```python
from build123d import *

# Parameters (mm, degrees)
F1_DEPTH = 39.6875
F2_W     = 152.4
F2_H     = 25.4
F3_DEPTH = 42.8625
F4_W     = 152.4
F4_H     = 13.716
F5_DEPTH = 42.8498


with BuildPart() as f1:
    # F0 (on Front) → F1 (new body)
    with BuildSketch(Plane.XZ):
        with BuildLine():
            Line((0, 25.4), (0, 0))
            Line((0, 0), (34.078865, 0))
            ThreePointArc((34.078865, 0), (76.2, 12.7), (118.321135, 0))
            Line((118.321135, 0), (152.4, 0))
            Line((152.4, 0), (152.4, 25.4))
            Line((152.4, 25.4), (0, 25.4))
        make_face()
    extrude(amount=F1_DEPTH)

    # F2 (on face) → F3 (join)
    with BuildSketch(Plane(origin=(0, 0, 0), x_dir=(-1, 0, 0), z_dir=(0, 1, 0))):
        with Locations((-76.2, 12.7)):
            Rectangle(F2_W, F2_H)
    extrude(amount=F3_DEPTH)

    # F4 (on face) → F5 (cut)
    with BuildSketch(Plane(origin=(0, 42.8625, 0), x_dir=(-1, 0, 0), z_dir=(0, 1, 0))):
        with Locations((-76.2, 18.542)):
            Rectangle(F4_W, F4_H)
    extrude(amount=-F5_DEPTH, mode=Mode.SUBTRACT)


solid = f1.part
```
The listing builds one solid part. Answer for the finished solid, in the listing's coordinates (mm). A direction names the side the tool comes from. Give positions to 0.01 mm unless a question says otherwise; leave off trailing zeros. Order: outer loops, then holes, each group sorted by start corner. A loop starts at its lowest first (then second) coordinate and runs counter-clockwise, first axis right, second up.
Item 1: For a pull along X with two mould halves and no side action, classify faces 1 (the face through (75.575, -19.566, 12.697)), 2 (the face through (77, 0.013, 19)), 3 (the face through (152.4, -8, 10)) as pulls with the +X half, pulls with the -X half, needs draft (parallel to the pull), parting line crosses it, or undercut.
From the geometry:
face 1: undercut
face 2: needs draft
face 3: pulls with the +X half
Item 2: The part is cut by section A-A, the plane y = -8. Give the vertices of the cut face in (x, z), and give its area (3 significant figures).
From the geometry:
outline: (0, 0) - (34.08, 0) arc R76.2 cw to (118.32, 0) - (152.4, 0) - (152.4, 25.4) - (0, 25.4) - close
area: 3,140 mm2
Item 3: The part is cut by section C-C, the plane z = 3.5. Give the vertices of the cut face in (x, y), and give its area (3 significant figures).
From the geometry:
outline: (0, -39.69) - (39.9, -39.69) - (39.9, 0) - (112.5, 0) - (112.5, -39.69) - (152.4, -39.69) - (152.4, 42.86) - (0, 42.86) - close
area: 9,700 mm2
Item 4: Given pin 1 Ø2 at (x, y) = (82, 9.5) entering from +Z; pin 2 Ø4 at (x, z) = (61, 5.5) entering from -Y, each flat-ended and moving along its own axis, determine where each tip first touches the part or whether it passes through.
From the geometry:
pin 1: stops at z = 11.68
pin 2: stops at y = 0
Item 5: The part is cut by section D-D, the plane x = 132.5. Give the vertices of the cut face in (y, z), and give its area (3 significant figures).
From the geometry:
outline: (-39.69, 0) - (42.86, 0) - (42.86, 11.68) - (0.01, 11.68) - (0.01, 25.4) - (-39.69, 25.4) - close
area: 1,510 mm2
Item 6: Find the intervals of material crossed by probe 1 along Y at (x, z) = (26, 12.75); probe 2 along Z at (x, y) = (96, 17); probe 3 along Z at (x, y) = (53, -34), in increasing order.
From the geometry:
probe 1: y = -39.69 to 0.01
probe 2: z = 0 to 11.68
probe 3: z = 9.08 to 25.4
Item 7: The part is cut by section B-B, the plane x = 49. Give the vertices of the cut face in (y, z), and give its area (3 significant figures).
From the geometry:
outline: (-39.69, 7.68) - (0, 7.68) - (0, 0) - (42.86, 0) - (42.86, 11.68) - (0.01, 11.68) - (0.01, 25.4) - (-39.69, 25.4) - close
area: 1,200 mm2
Item 8: Which of the six approach directions +Z, -Z, +X, -X, +Y, -Y give full straight-line access (tool end or side, diameter ignored) to faces 4 (the face through (77, 0, 5)), 5 (the face through (75, -39.688, 16)), 6 (the face through (77, 22, 11.684))?
From the geometry:
face 4: -Z, -Y
face 5: +Z, -Z, +X, -X, -Y
face 6: +Z, +X, -X, +Y
